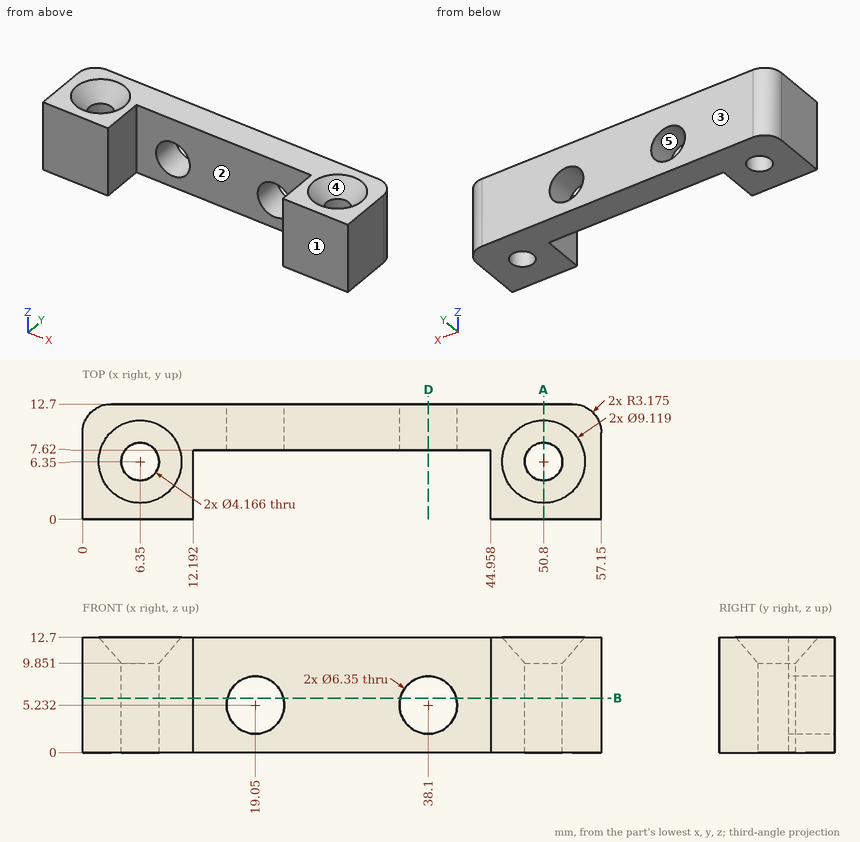
Design review of the part shown in the three views and the two pictorial views. Dimensions are in mm from the part's minimum x, y and z. A direction names the side the tool comes from. Coordinates: 2 decimals unless noted, no trailing zeros. Order: outer loops, then holes, each group sorted by start corner. A loop starts at its lowest first (then second) coordinate and runs counter-clockwise, first axis right, second up.
Item 1: Take a section at D-D, the plane x = 38.1. Write out the cut boundary in (y, z).
Item 2: Take a section at B-B, the plane z = 6. Count the separate pieces of the cut face and the enclosed holes in it, then the cut area to 3 significant figures.
Item 3: The part is to be moulded in two halves that separate along Y. For the marked faces 3, 4 and 5, say which applies: pulls with the +Y half, pulls with the -Y half, needs draft (parallel to the pull), parting line crosses it, or undercut.
Item 4: For line 1 (X direction, y = 6.35, z = 7.5); line 2 (X direction, y = 3, z = 1.5); line 3 (X direction, y = 8.5, z = 4.25), list the stretches that pass through material, from the lowest coordinate up.
Item 5: For pin 1 Ø6 at (x, z) = (40.5, 2.5) entering from -Y, flat-tipped, find the tip position at first contact; note if it passes through.
Item 6: For the marked faces 1 and 2, list the 3-axis set-ups (+Z, -Z, +X, -X, +Y, -Y) from which the entire face can be reached by the end or side of a thin tool; tool diameter is ignored.
Item 7: Take a section at A-A, the plane x = 50.8. Write out the cut boundary in (y, z), then the cut area to 3 significant figures.
The answers:
1. outline: (7.62, 0) - (12.7, 0) - (12.7, 2.06) - (7.62, 2.06) - close; (7.62, 8.41) - (12.7, 8.41) - (12.7, 12.7) - (7.62, 12.7) - close
2. separate pieces: 3
2. enclosed holes: 2
2. area: 382 mm2
3. face 3: pulls with the +Y half
3. face 4: undercut
3. face 5: needs draft
4. line 1: x = 0 to 4.27, 8.43 to 12.19, 44.96 to 48.72, 52.88 to 57.15
4. line 2: x = 0 to 12.19, 44.96 to 57.15
4. line 3: x = 0 to 16.03, 22.07 to 35.08, 41.12 to 57.15
5. pin 1: stops at y = 7.62
6. face 1: +Z, -Z, +X, -X, -Y
6. face 2: +Z, -Z, -Y
7. outline: (0, 0) - (4.27, 0) - (4.27, 9.85) - (1.79, 12.7) - (0, 12.7) - close; (8.43, 0) - (12.7, 0) - (12.7, 12.7) - (10.91, 12.7) - (8.43, 9.85) - close
7. area: 101 mm2
